Verification items for the finished model (mm, model axes). Face numbers are marked on the shaded views. A direction names the side the tool comes from. Coordinates: 2 decimals unless noted, no trailing zeros. Order: outer loops, then holes, each group sorted by start corner. A loop starts at its lowest first (then second) coordinate and runs counter-clockwise, first axis right, second up. Notation, with made-up numbers: M 73,-8.5 L 92,-8.5 A17 cw 92,-3.5 Z; hole C 64.5,-31.5 d10. An arc over 180 degrees is marked long. Return JSON: item names as keys, results as strings.
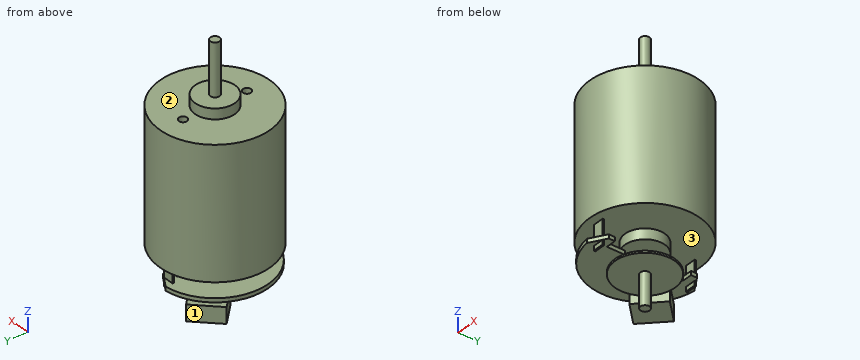
```python
from build123d import *

# Parameters (mm, degrees)
MAINBODY_DEPTH               = 16.3
MAINBODY_DEPTH_BACK          = 16.3
SKETCH1_R                    = 13.85
SKETCH2_R                    = 1.15
OUTPUTSHAFT_DEPTH            = 15.6
SKETCH2_3_R                  = 5
SKETCH2_3_R_2                = 1.15
OUTPUTBOSS_DEPTH             = 2.6
M2_5X0_45_TAPPED_HOLE1_D     = 2.05
M2_5X0_45_TAPPED_HOLE1_DEPTH = 6.35
M2_5X0_45_TAPPED_HOLE1_TIP   = 0.615882135
SKETCH5_W                    = 2.8
SKETCH5_H                    = 0.4
TERMINALS_DEPTH              = 6.1
PCB_START                    = 4
PCB_DEPTH                    = 1
ENCODER_START                = 7
SKETCH9_R                    = 7.5
ENCODER_DEPTH                = 0.5
CONNECTOR_DEPTH              = 4


with BuildPart() as part:
    # Sketch1 → MAINBODY (new, two sides: drawn at the far end of the back side and taken through both)
    with BuildSketch(Plane.XY.offset(-MAINBODY_DEPTH_BACK)):
        Circle(SKETCH1_R)
    extrude(amount=MAINBODY_DEPTH + MAINBODY_DEPTH_BACK)

    # Sketch2 → OUTPUTSHAFT (add)
    with BuildSketch(Plane.XY.offset(16.3)):
        Circle(SKETCH2_R)
    outputshaft = extrude(amount=OUTPUTSHAFT_DEPTH)

    # Sketch2<3> → OUTPUTBOSS (add)
    with BuildSketch(Plane.XY.offset(16.3)):
        Circle(SKETCH2_3_R)
        Circle(SKETCH2_3_R_2, mode=Mode.SUBTRACT)
    outputboss = extrude(amount=OUTPUTBOSS_DEPTH)

    # M2.5x0.45 Tapped Hole1
    with Locations(Plane.XY.offset(16.3)):
        with Locations((0, 8), (0, -8)):
            Hole(M2_5X0_45_TAPPED_HOLE1_D / 2, depth=M2_5X0_45_TAPPED_HOLE1_DEPTH)
            with Locations((0, 0, -(M2_5X0_45_TAPPED_HOLE1_DEPTH + M2_5X0_45_TAPPED_HOLE1_TIP / 2))):  # 118° drill point
                Cone(0, M2_5X0_45_TAPPED_HOLE1_D / 2, M2_5X0_45_TAPPED_HOLE1_TIP, mode=Mode.SUBTRACT)

    # REARSHAFT: OUTPUTSHAFT, OUTPUTBOSS across plane
    add(outputshaft.mirror(Plane.XY))
    add(outputboss.mirror(Plane.XY))

    # Sketch5 → TERMINALS (add)
    with BuildSketch(Plane(origin=(0, 0, -16.3), x_dir=(-1, 0, 0), z_dir=(0, 0, -1))):
        with Locations((0, 11.5)):
            Rectangle(SKETCH5_W, SKETCH5_H)
        with Locations((0, -11.5)):
            Rectangle(SKETCH5_W, SKETCH5_H)
    extrude(amount=TERMINALS_DEPTH)

    # Sketch8 → PCB (add)
    with BuildSketch(Plane(origin=(0, 0, -16.3), x_dir=(-1, 0, 0), z_dir=(0, 0, -1)).offset(PCB_START)):
        with BuildLine():
            Line((1.4, 13.427211177), (-2.5, 11.021452752))
            Line((-2.5, 11.021452752), (-2.5, 9.521452752))
            Line((-2.5, 9.521452752), (0, 9.521452752))
            Line((0, 9.521452752), (0, 5))
            ThreePointArc((0, 5), (5, 0), (0, -5))
            Line((0, -5), (0, -9.521452752))
            Line((0, -9.521452752), (-2.5, -9.521452752))
            Line((-2.5, -9.521452752), (-2.5, -11.021452752))
            Line((-2.5, -11.021452752), (1.4, -13.427211177))
            ThreePointArc((1.4, -13.427211177), (13.5, 0), (1.4, 13.427211177))
        make_face()
    extrude(amount=PCB_DEPTH)

    # Sketch9 → ENCODER (add)
    with BuildSketch(Plane(origin=(0, 0, -16.3), x_dir=(-1, 0, 0), z_dir=(0, 0, -1)).offset(ENCODER_START)):
        Circle(SKETCH9_R)
    extrude(amount=ENCODER_DEPTH)

    # Sketch10 → CONNECTOR (add)
    with BuildSketch(Plane(origin=(0, 0, -21.3), x_dir=(-1, 0, 0), z_dir=(0, 0, -1))):
        Polygon((2.651397898, 8.308757211), (8.308252147, 2.651902961), (13.257999616, 7.601650429), (7.601145366, 13.258504679), align=None)
    extrude(amount=CONNECTOR_DEPTH)


solid = part.part
```
Q1. Cross-section at C-C, the plane y = -6.25. Record the boundary of the cut face in (x, z), and give its area (3 significant figures).
Values:
{"outline": "M -12.36,-16.3 L 12.36,-16.3 L 12.36,16.3 L -12.36,16.3 Z; M -11.97,-21.3 L 0,-21.3 L 0,-20.3 L -11.97,-20.3 Z; M -4.15,-23.8 L 4.15,-23.8 L 4.15,-23.3 L -4.15,-23.3 Z", "area": "822 mm^2"}
Q2. Tool access check on the marked faces 1, 2 and 3. Record the directions out of +Z, -Z, +X, -X, +Y, -Y that give a thin tool (end or side, any length) a straight path to the whole face; none if there is none.
Values:
{"face 1": "+Z, -Z, -X, +Y", "face 2": "+Z", "face 3": "none"}
Q3. Go/stop test with flat-tipped pins: pin 1 (7.5 mm diameter, centred on x = -9, y = 8, fed in from +Z); pin 2 (2 mm diameter, centred on x = -2, y = 1, fed in from +Z); pin 3 (1.4 mm diameter, centred on x = -0.5, z = -18.5, fed in from -Y). Record where each tip stops, or that it passes through.
Values:
{"pin 1": "z = 16.3", "pin 2": "z = 18.9", "pin 3": "y = -11.7"}
Q4. Material ranges on line 1 along Y through (x, z) = (0, 12.25) (3 decimals); line 2 along Z through (x, y) = (-6.25, 4); line 3 along Z through (x, y) = (-12.25, 0.75), recorded low to high.
Values:
{"line 1": "-13.85 to -9.025, -6.975 to 6.975, 9.025 to 13.85", "line 2": "-23.8 to -23.3, -21.3 to -20.3, -16.3 to 16.3", "line 3": "-21.3 to -20.3, -16.3 to 16.3"}
Q5. Cross-section at B-B, the plane x = 6.5. Record the boundary of the cut face in (y, z).
Values:
{"outline": "M -12.23,-16.3 L 12.23,-16.3 L 12.23,16.3 L -12.23,16.3 Z; M -3.74,-23.8 L 3.74,-23.8 L 3.74,-23.3 L -3.74,-23.3 Z"}
Q6. Cross-section at D-D, the plane z = 19.5. Record the boundary of the cut face in (x, y), and give its area (3 significant figures).
Values:
{"outline": "C 0,0 d2.3", "area": "4.15 mm^2"}
